Verification items for the finished model (mm, model axes). A direction names the side the tool comes from. Give positions to 0.01 mm unless a question says otherwise; leave off trailing zeros. Write each loop counter-clockwise with the first axis right and the second up, starting at its lowest first coordinate (ties: lowest second). Pieces come first, ordered by that corner, then holes. Notation, with made-up numbers: (4, -26) - (26, -26) arc R36 ccw to (26, 13) - close; hole circle Ø8 at (-1, 54). An arc over 180 degrees is marked (long way). Put each result on its own line as item: value.
from build123d import *

# Parameters (mm, degrees)
SKETCH1_R               = 10
BOSS_EXTRUDE1_DEPTH     = 13.4
SKETCH2_R               = 14.5
BOSS_EXTRUDE2_DEPTH     = 3
SKETCH3_R               = 4.7625
CUT_EXTRUDE1_DEPTH      = 16.4
CUT_EXTRUDE2_REACH      = 28.258
CUT_EXTRUDE2_END_RADIUS = 10
SKETCH4_R               = 1.89865


with BuildPart() as part:
    # Sketch1 → Boss-Extrude1 (new body)
    with BuildSketch(Plane.XY):
        Circle(SKETCH1_R)
    extrude(amount=BOSS_EXTRUDE1_DEPTH)

    # Sketch2 → Boss-Extrude2 (add)
    with BuildSketch(Plane.XY.offset(13.4)):
        Circle(SKETCH2_R)
    extrude(amount=BOSS_EXTRUDE2_DEPTH)

    # Sketch3 → Cut-Extrude1 (cut)
    with BuildSketch(Plane.XY.offset(16.4)):
        Circle(SKETCH3_R)
    extrude(amount=-CUT_EXTRUDE1_DEPTH, mode=Mode.SUBTRACT)

    # Cut-Extrude2: up to this cylinder (the profile starts inside it)
    cut_extrude2_end = Plane(origin=(0, 0, 5), z_dir=(0, 0, -1)) * Cylinder(CUT_EXTRUDE2_END_RADIUS, 77.516, mode=Mode.PRIVATE)
    # Sketch4 → Cut-Extrude2 (cut, up to the surface)
    with BuildSketch(Plane(origin=(0, 0, 0), x_dir=(0, 0, -1), z_dir=(1, 0, 0)), mode=Mode.PRIVATE) as cut_extrude2_sk1:
        with Locations((-5, 0)):
            Circle(SKETCH4_R)
    cut_extrude2_tool1 = extrude(cut_extrude2_sk1.sketch, amount=-CUT_EXTRUDE2_REACH, mode=Mode.PRIVATE) & cut_extrude2_end
    add(cut_extrude2_tool1.solids().sort_by_distance((0, 0, 5))[0], mode=Mode.SUBTRACT)


solid = part.part
Q1. Set-up check for faces 1 (the face through (9.54, 3, 6.61)), 2 (the face through (-2.4, -4.3, 0)): record each of +Z, -Z, +X, -X, +Y, -Y from which the full face is reachable in a straight line by a thin tool's end or side.
Answers follow:
face 1: -Z
face 2: -Z, +X, -X, +Y, -Y
Q2. Scan lines: line 1 along X through (y, z) = (3, 7.5); line 2 along Z through (x, y) = (-10.5, -1); line 3 along X through (y, z) = (-4, 15.25). Record each from-to range of solid material in increasing order.
Answers follow:
line 1: x = -9.54 to -3.7, 3.7 to 9.54
line 2: z = 13.4 to 16.4
line 3: x = -13.94 to -2.58, 2.58 to 13.94
Q3. Section check A-A, the plane x = 0. Record the cut outline in (y, z), plus the area to 3 significant figures.
Answers follow:
outline: (-14.5, 13.4) - (-10, 13.4) - (-10, 0) - (-4.76, 0) - (-4.76, 16.4) - (-14.5, 16.4) - close; (4.76, 0) - (10, 0) - (10, 13.4) - (14.5, 13.4) - (14.5, 16.4) - (4.76, 16.4) - close
area: 199 mm2
Q4. Go/stop test with flat-tipped pins: pin 1 Ø8 at (y, z) = (6, 6) entering from -X; pin 2 Ø5 at (y, z) = (-9, 12) entering from +X; pin 3 Ø8 at (x, z) = (-5, 2) entering from +Y. Record where each tip stops, or that it passes through.
Answers follow:
pin 1: stops at x = -9.8
pin 2: stops at x = 12.74
pin 3: stops at y = 9.95
Q5. Release check for a two-part mould opening along Z. For faces 3 (the face through (6.691, -12.864, 14.879)), 4 (the face through (-7.145, 0.083, 6.897)), 5 (the face through (6, 0, 16.4)), 6 (the face through (3, 10, 13.4)) record: released by +Z, released by -Z, zero draft, split by the parting line, or undercut.
Answers follow:
face 3: zero draft
face 4: undercut
face 5: released by +Z
face 6: released by -Z
Q6. Section check D-D, the plane y = -5.5. Record the cut outline in (x, z), plus the area to 3 significant figures.
Answers follow:
outline: (-13.42, 13.4) - (-8.35, 13.4) - (-8.35, 0) - (8.35, 0) - (8.35, 13.4) - (13.42, 13.4) - (13.42, 16.4) - (-13.42, 16.4) - close
area: 304 mm2
Q7. Section check C-C, the plane z = 14.25. Record the cut outline in (x, y) (1 decimal), plus the area to 3 significant figures.
Answers follow:
outline: circle Ø29 at (0, 0); hole circle Ø9.5 at (0, 0)
area: 589 mm2
Q8. Section check B-B, the plane y = 0. Record the cut outline in (x, z), plus the area to 3 significant figures.
Answers follow:
outline: (-14.5, 13.4) - (-10, 13.4) - (-10, 6.9) - (-4.76, 6.9) - (-4.76, 16.4) - (-14.5, 16.4) - close; (-10, 0) - (-4.76, 0) - (-4.76, 3.1) - (-10, 3.1) - close; (4.76, 0) - (10, 0) - (10, 13.4) - (14.5, 13.4) - (14.5, 16.4) - (4.76, 16.4) - close
area: 179 mm2
